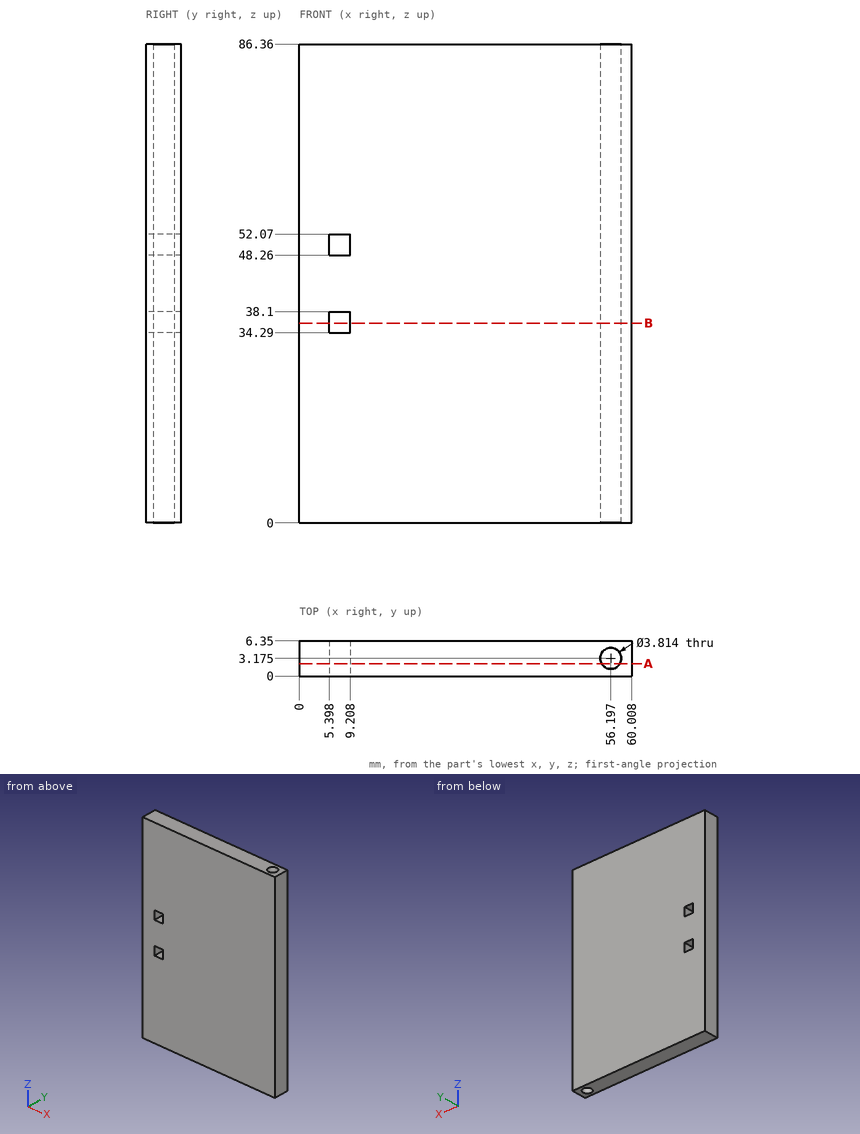
Input: dimensioned drawing with shaded views. Units: mm. Origin: part minimum x, y, z. Give positions to 0.01 mm unless a question says otherwise; leave off trailing zeros. Write each loop counter-clockwise with the first axis right and the second up, starting at its lowest first coordinate (ties: lowest second). Pieces come first, ordered by that corner, then holes. Notation, with made-up numbers: M 58.25,-30 L 105.25,-30 A7 ccw 105.25,-18 Z; hole C 74.5,-38 d3. An arc over 180 degrees is marked long. Write item = value, one per line. Start each with the question number.
1) Cut plane A-A on y = 2.25. Return the cut outline in (x, z) (1 decimal).
2) Cut plane B-B on z = 36. Count the separate pieces of the cut face and the enclosed holes in it.
3) Material intervals for line 1 along Z through (x, y) = (7, 5.25); line 2 along X through (y, z) = (2.5, 49) (1 decimal); line 3 along X through (y, z) = (3.5, 68.5), sorted ascending. Write a range as [from, to].
Solved:
q1.outline = M 0,0 L 54.5,0 L 54.5,86.4 L 0,86.4 Z; M 57.9,0 L 60,0 L 60,86.4 L 57.9,86.4 Z; hole M 5.4,34.3 L 9.2,34.3 L 9.2,38.1 L 5.4,38.1 Z; hole M 5.4,48.3 L 9.2,48.3 L 9.2,52.1 L 5.4,52.1 Z
q2.separate_pieces = 2
q2.enclosed_holes = 1
q3.line_1 = [0, 34.29], [38.1, 48.26], [52.07, 86.36]
q3.line_2 = [0, 5.4], [9.2, 54.4], [58, 60]
q3.line_3 = [0, 54.32], [58.08, 60.01]
